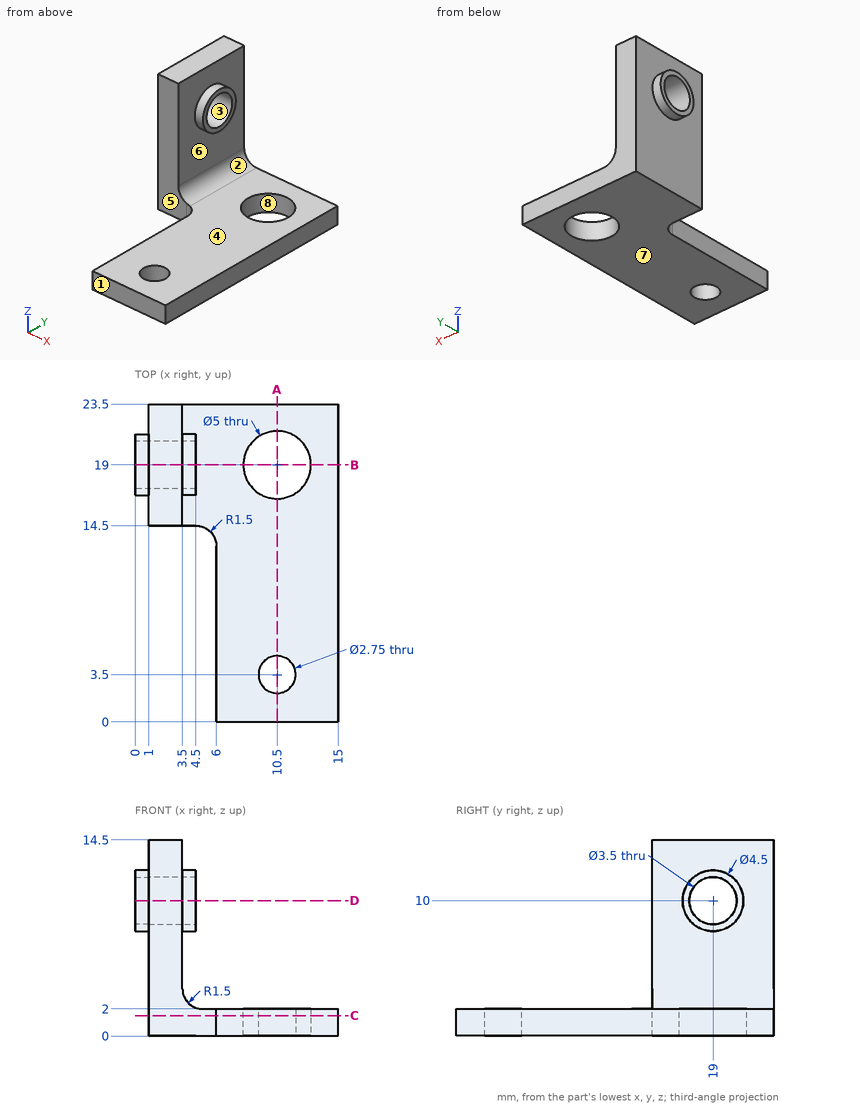
Study the drawing (mm; zero at the part's minimum x, y, z) and answer. A direction names the side the tool comes from. Round coordinates to 2 decimals unless told otherwise and drop trailing zeros. Write each loop counter-clockwise with the first axis right and the second up, starting at its lowest first coordinate (ties: lowest second). Pieces come first, ordered by that corner, then holes. Notation, with made-up numbers: (57.5, -15) - (96.5, -15) arc R28 ccw to (96.5, 21) - close; hole circle Ø9 at (49.5, 30). An arc over 180 degrees is marked (long way). Return JSON: item names as keys, results as strings. Group by question number.
Q1. Each of these flat-tipped pins is pushed along its axis until it touches: pin 1 Ø4.5 at (y, z) = (19, 10) entering from -X; pin 2 Ø8 at (x, y) = (12.5, 9) entering from +Z; pin 3 Ø1 at (x, z) = (2, 9.5) entering from -Y; pin 4 Ø5 at (y, z) = (18, 10.5) entering from +X. Where does it stop, or does it pass through?
Q2. Find the intervals of material crossed by L1, parallel to Y at x = 10.5, z = 1.2 (3 decimals); L2, parallel to Y at x = 1.9, z = 10; L3, parallel to Z at x = 1.9, y = 19, in increasing order.
Q3. For the marked faces 1, 2, 3, 4 and 5, determine the directions among +Z, -Z, +X, -X, +Y, -Y from which every point of the face is accessible in a straight line to the end or side of a thin tool.
Q4. The mould has two halves that part along Z. Classify the marked faces 6, 7 and 8: released by +Z, released by -Z, zero draft, split by the parting line, or undercut.
Q5. The part is cut by section D-D on z = 10. Write down the section's boundary in (x, y).
Q6. The part is cut by section C-C on z = 1.5. Write down the section's boundary in (x, y) (3 decimals), then the cut area to 3 significant figures.
Q7. The part is cut by section A-A on x = 10.5. Write down the section's boundary in (y, z) (3 decimals), then the cut area to 3 significant figures.
Q8. The part is cut by section B-B on y = 19. Write down the section's boundary in (x, z), then the cut area to 3 significant figures.
Solved:
{
 "1": {"pin 1": "x = 0", "pin 2": "z = 2", "pin 3": "y = 14.5", "pin 4": "x = 4.5"},
 "2": {"L1": "0 to 2.125, 4.875 to 16.5, 21.5 to 23.5", "L2": "14.5 to 17.25, 20.75 to 23.5", "L3": "0 to 8.25, 11.75 to 14.5"},
 "3": {"face 1": "+Z, -Z, +X, -X, -Y", "face 2": "+X, +Y, -Y", "face 3": "+X, -X", "face 4": "+Z, +X, +Y, -Y", "face 5": "+Z, -Z, -X, -Y"},
 "4": {"face 6": "undercut", "face 7": "released by -Z", "face 8": "zero draft"},
 "5": {"outline": "(0, 16.75) - (1, 16.75) - (1, 14.5) - (3.5, 14.5) - (3.5, 16.75) - (4.5, 16.75) - (4.5, 17.25) - (0, 17.25) - close; (0, 20.75) - (4.5, 20.75) - (4.5, 21.25) - (3.5, 21.25) - (3.5, 23.5) - (1, 23.5) - (1, 21.25) - (0, 21.25) - close"},
 "6": {"outline": "(1, 14.5) - (4.5, 14.5) arc R1.5 cw to (6, 13) - (6, 0) - (15, 0) - (15, 23.5) - (1, 23.5) - close; hole circle Ø5 at (10.5, 19); hole circle Ø2.75 at (10.5, 3.5)", "area": "231 mm²"},
 "7": {"outline": "(0, 0) - (2.125, 0) - (2.125, 2) - (0, 2) - close; (4.875, 0) - (16.5, 0) - (16.5, 2) - (4.875, 2) - close; (21.5, 0) - (23.5, 0) - (23.5, 2) - (21.5, 2) - close", "area": "31.5 mm²"},
 "8": {"outline": "(0, 7.75) - (1, 7.75) - (1, 0) - (8, 0) - (8, 2) - (5, 2) arc R1.5 cw to (3.5, 3.5) - (3.5, 7.75) - (4.5, 7.75) - (4.5, 8.25) - (0, 8.25) - close; (0, 11.75) - (4.5, 11.75) - (4.5, 12.25) - (3.5, 12.25) - (3.5, 14.5) - (1, 14.5) - (1, 12.25) - (0, 12.25) - close; (13, 0) - (15, 0) - (15, 2) - (13, 2) - close", "area": "43.0 mm²"}
}
